Source: CAD feature listing. Evaluate the final solid. Frame: model axes, mm. A direction names the side the tool comes from. Round coordinates to 2 decimals unless told otherwise and drop trailing zeros. Loops run counter-clockwise (first coordinate to the right, second up) from the corner with the lowest first, then second, coordinate; pieces in that order, holes last. Notation, with made-up numbers: M 53,-15 L 87,-15 A18 ccw 87,-6 Z; hole C 8,-32.5 d6. An arc over 180 degrees is marked long. Answer as a JSON object with one key per item and string values.
from build123d import *

# Parameters (mm, degrees)
SKETCH1_W           = 7.366
SKETCH1_H           = 7.366
BOSS_EXTRUDE1_DEPTH = 33.02
SKETCH2_R           = 13.335
CUT_EXTRUDE1_DEPTH  = 3.81
FILLET1_R           = 12.7


with BuildPart() as part:
    # Sketch1 → Boss-Extrude1 (new body)
    with BuildSketch(Plane.XY):
        Polygon((48.76226865, 0), (41.39626865, 0), (13.20226865, 0), (13.20226865, 6.709268486), (114.80226865, 6.709268486), (114.80226865, 0), (86.60826865, 0), (79.24226865, 0), align=None)
        with Locations((45.07926865, -3.683)):
            Rectangle(SKETCH1_W, SKETCH1_H)
        with Locations((82.92526865, -3.683)):
            Rectangle(SKETCH1_W, SKETCH1_H)
    extrude(amount=BOSS_EXTRUDE1_DEPTH)

    # Sketch2 → Cut-Extrude1 (cut)
    with BuildSketch(Plane(origin=(0, 6.709268486, 0), x_dir=(1, 0, 0), z_dir=(0, 1, 0))):
        with Locations((38.60226865, -16.51)):
            Circle(SKETCH2_R)
        with Locations((89.40226865, -16.51)):
            Circle(SKETCH2_R)
    extrude(amount=-CUT_EXTRUDE1_DEPTH, mode=Mode.SUBTRACT)

    # Fillet1
    fillet1_edges = [part.edges().sort_by_distance(p)[0] for p in [
        (114.80226865, 3.354634243, 33.02),
        (13.20226865, 3.354634243, 0),
        (114.80226865, 3.354634243, 0),
        (13.20226865, 3.354634243, 33.02),
    ]]
    fillet(fillet1_edges, radius=FILLET1_R)


solid = part.part
Item 1: Section D-D on x = 91. Return the cut outline in (y, z).
Answer sheet:
{"outline": "M 0,0 L 6.71,0 L 6.71,3.27 L 2.9,3.27 L 2.9,29.75 L 6.71,29.75 L 6.71,33.02 L 0,33.02 Z"}
Item 2: Contact query for flat-ended pins moving along their axis: pin 1 Ø3.5 at (y, z) = (-3, 9.5) entering from +X; pin 2 Ø8.5 at (x, z) = (33.5, 10.5) entering from -Y; pin 3 Ø6 at (y, z) = (-2.5, 10) entering from +X; pin 4 Ø6 at (y, z) = (-2, 19) entering from -X. Output: stop coordinate, or through.
Answer sheet:
{"pin 1": "stops at x = 86.61", "pin 2": "stops at y = 0", "pin 3": "stops at x = 114.76", "pin 4": "stops at x = 13.2"}
Item 3: Line query: probe 1 along X at (y, z) = (5.85, 16.51); probe 2 along X at (y, z) = (-6, 21); probe 3 along Z at (x, y) = (38, 4.75). Output: solid intervals per line, ascending. Write a range as from..to.
Answer sheet:
{"probe 1": "x = 13.2..25.27, 51.94..76.07, 102.74..114.8", "probe 2": "x = 41.4..48.76, 79.24..86.61", "probe 3": "z = 0..3.19, 29.83..33.02"}
Item 4: Pull-direction query (Z, two-part tool) for faces 5 (the flat face through (48.762, -4, 16)), 6 (the flat face through (89, 2.899, 16)), 7 (the cylindrical face through (50.92, 4.83, 21.62)), 8 (the cylindrical face through (16.824, 3.402, 3.819)); classes: pulls with the +Z half, pulls with the -Z half, needs draft (parallel to the pull), parting line crosses it, or undercut.
Answer sheet:
{"face 5": "needs draft", "face 6": "undercut", "face 7": "undercut", "face 8": "pulls with the -Z half"}
Item 5: Section A-A on y = -2. Return the cut outline in (x, z).
Answer sheet:
{"outline": "M 41.4,0 L 48.76,0 L 48.76,33.02 L 41.4,33.02 Z; M 79.24,0 L 86.61,0 L 86.61,33.02 L 79.24,33.02 Z"}
Item 6: Access query for faces 1 (the flat face through (27, 0, 16)), 2 (the cylindrical face through (101.72, 4.83, 21.62)), 3 (the flat face through (64, 0, 16)), 4 (the flat face through (101, 0, 16)). Directions: +Z, -Z, +X, -X, +Y, -Y. A direction counts if a zero-diameter tool reaches every point of the face in a straight line with its end or side. Return the directions, or none.
Answer sheet:
{"face 1": "+Z, -Z, -X, -Y", "face 2": "+Y", "face 3": "+Z, -Z, -Y", "face 4": "+Z, -Z, +X, -Y"}
Item 7: Section B-B on z = 16.51. Return the cut outline in (x, y).
Answer sheet:
{"outline": "M 13.2,0 L 41.4,0 L 41.4,-7.37 L 48.76,-7.37 L 48.76,0 L 79.24,0 L 79.24,-7.37 L 86.61,-7.37 L 86.61,0 L 114.8,0 L 114.8,6.71 L 102.74,6.71 L 102.74,2.9 L 76.07,2.9 L 76.07,6.71 L 51.94,6.71 L 51.94,2.9 L 25.27,2.9 L 25.27,6.71 L 13.2,6.71 Z"}
Item 8: Section C-C on x = 32.5. Return the cut outline in (y, z), then the cut area to 3 significant figures.
Answer sheet:
{"outline": "M 0,0 L 6.71,0 L 6.71,4.65 L 2.9,4.65 L 2.9,28.37 L 6.71,28.37 L 6.71,33.02 L 0,33.02 Z", "area": "131 mm²"}
